Build history of the part. All positions in model axes, mm. Face numbers are marked on the shaded views. A direction names the side the tool comes from. Round coordinates to 2 decimals unless told otherwise and drop trailing zeros. Write each loop counter-clockwise with the first axis right and the second up, starting at its lowest first coordinate (ties: lowest second). Pieces come first, ordered by that corner, then holes.
1) Which spindle directions (+Z, -Z, +X, -X, +Y, -Y) get a long thin tool onto all of the face, cutting with end or side? Do the marked faces 1 and 2. Say none if no direction does.
2) Saw through at B-B (x = 0). Write the cut outline in (y, z), plus the area to 3 significant figures.
3) Saw through at C-C (z = 4.2). Write the cut outline in (x, y), plus the area to 3 significant figures.
4) Saw through at D-D (y = 4.5). Write the cut outline in (x, z), plus the area to 3 significant figures.
5) Wall check: probe 1 along X at (y, z) = (0, 6.25); probe 2 along Z at (x, y) = (-5.8, 0); probe 3 along X at (y, z) = (2, 7.75). Give the ranges that are in metal, low to high.
6) Pull direction X, two halves, no side cores. Call the marked faces 3, 4 and 5: +X half, -X half, draft (parallel to the pull), parting line (faces both ways), or undercut.
7) Saw through at A-A (y = 0). Write the cut outline in (x, z), plus the area to 3 significant figures.
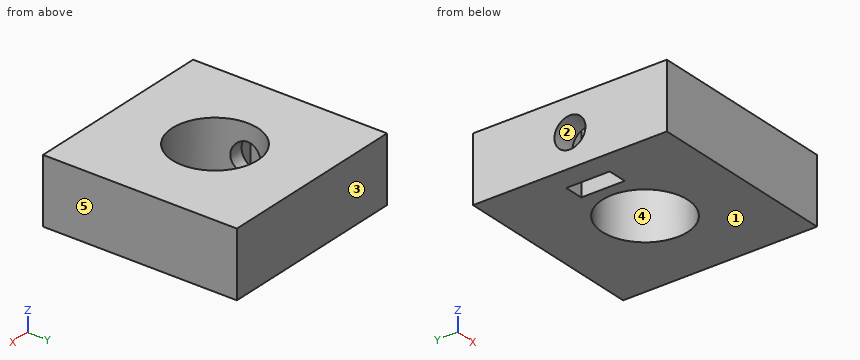
from build123d import *

# Parameters (mm, degrees)
SKETCH002_W      = 2.5
SKETCH002_H      = 5.6
EXTRUDE002_DEPTH = 8.2
SKETCH001_R      = 2
EXTRUDE001_DEPTH = 20
SKETCH_W         = 25
SKETCH_H         = 25
SKETCH_R         = 5.5
EXTRUDE_DEPTH    = 8.4


with BuildPart() as extrude002:
    # Sketch002 → Extrude002 (new body)
    with BuildSketch(Plane.XY):
        with Locations((-8.25, 0)):
            Rectangle(SKETCH002_W, SKETCH002_H)
    extrude(amount=EXTRUDE002_DEPTH)


with BuildPart() as extrude001:
    # Sketch001 → Extrude001 (new body)
    with BuildSketch(Plane.YZ):
        with Locations((0, 4.2)):
            Circle(SKETCH001_R)
    extrude(amount=-EXTRUDE001_DEPTH)


with BuildPart() as body:
    # Sketch → Extrude (new body)
    with BuildSketch(Plane.XY):
        Rectangle(SKETCH_W, SKETCH_H)
        Circle(SKETCH_R, mode=Mode.SUBTRACT)
    extrude(amount=EXTRUDE_DEPTH)

    # Cut: cut Extrude001
    add(extrude001.part, mode=Mode.SUBTRACT)

    # Cut001: cut Extrude002
    add(extrude002.part, mode=Mode.SUBTRACT)


solid = body.part
Evaluation:
1. face 1: -Z, +X, -X, +Y, -Y
1. face 2: -X
2. outline: (-12.5, 0) - (-5.5, 0) - (-5.5, 8.4) - (-12.5, 8.4) - close; (5.5, 0) - (12.5, 0) - (12.5, 8.4) - (5.5, 8.4) - close
2. area: 118 mm2
3. outline: (-12.5, -12.5) - (12.5, -12.5) - (12.5, 12.5) - (-12.5, 12.5) - (-12.5, 2) - (-9.5, 2) - (-9.5, 2.8) - (-7, 2.8) - (-7, 2) - (-5.12, 2) arc R5.5 cw (long way) to (-5.12, -2) - (-7, -2) - (-7, -2.8) - (-9.5, -2.8) - (-9.5, -2) - (-12.5, -2) - close
3. area: 497 mm2
4. outline: (-12.5, 0) - (-3.16, 0) - (-3.16, 8.4) - (-12.5, 8.4) - close; (3.16, 0) - (12.5, 0) - (12.5, 8.4) - (3.16, 8.4) - close
4. area: 157 mm2
5. probe 1: x = -12.5 to -9.5, -7 to -5.5, 5.5 to 12.5
5. probe 2: z = 0 to 2.2, 6.2 to 8.4
5. probe 3: x = -12.5 to -9.5, -7 to -5.12, 5.12 to 12.5
6. face 3: draft
6. face 4: undercut
6. face 5: +X half
7. outline: (-12.5, 0) - (-9.5, 0) - (-9.5, 2.2) - (-12.5, 2.2) - close; (-12.5, 6.2) - (-9.5, 6.2) - (-9.5, 8.2) - (-7, 8.2) - (-7, 6.2) - (-5.5, 6.2) - (-5.5, 8.4) - (-12.5, 8.4) - close; (-7, 0) - (-5.5, 0) - (-5.5, 2.2) - (-7, 2.2) - close; (5.5, 0) - (12.5, 0) - (12.5, 8.4) - (5.5, 8.4) - close
7. area: 79.1 mm2
